Work out the finished part from the listing and answer in its coordinate system (mm). A direction names the side the tool comes from. Round coordinates to 2 decimals unless told otherwise and drop trailing zeros. Order: outer loops, then holes, each group sorted by start corner. A loop starts at its lowest first (then second) coordinate and runs counter-clockwise, first axis right, second up. Notation, with made-up numbers: (83.25, 31.5) - (107.25, 31.5) arc R5 ccw to (107.25, 39.5) - close; hole circle Ø9 at (87, -24.75). An arc over 180 degrees is marked (long way). Answer in a Markdown table with one row per item.
from build123d import *

# Parameters (mm, degrees)
SKETCH1_W               = 21
SKETCH1_H               = 4
SKETCH1_W_2             = 4
SKETCH1_R               = 1.5
BOSS_EXTRUDE1_DEPTH     = 2
SKETCH1_3_W             = 21
SKETCH1_3_H             = 4
BOSS_EXTRUDE2_DEPTH     = 40
CUT_EXTRUDE1_DEPTH      = 50.568134926
CUT_EXTRUDE1_DEPTH_BACK = 50.568134926


with BuildPart() as part:
    # Sketch1 → Boss-Extrude1 (new body)
    # profile 1 of 3: a face of its own
    with BuildSketch(Plane(origin=(0, 0, 0), x_dir=(1, 0, 0), z_dir=(0, 1, 0))):
        with Locations((14.5, 2)):
            Rectangle(SKETCH1_W, SKETCH1_H)
    # profile 2 of 3: a face of its own
    with BuildSketch(Plane(origin=(0, 0, 0), x_dir=(1, 0, 0), z_dir=(0, 1, 0))):
        with Locations((2, 2)):
            Rectangle(SKETCH1_W_2, SKETCH1_H)
        with Locations(Location((1.985523286, 2, 0), (0, 0, 270))):
            Circle(SKETCH1_R, mode=Mode.SUBTRACT)
    # profile 3 of 3: a face of its own
    with BuildSketch(Plane(origin=(0, 0, 0), x_dir=(1, 0, 0), z_dir=(0, 1, 0))):
        with Locations((27, 2)):
            Rectangle(SKETCH1_W_2, SKETCH1_H)
        with Locations(Location((26.985523286, 2, 0), (0, 0, 270))):
            Circle(SKETCH1_R, mode=Mode.SUBTRACT)
    extrude(amount=BOSS_EXTRUDE1_DEPTH)

    # Sketch1_3 → Boss-Extrude2 (add)
    with BuildSketch(Plane(origin=(0, 0, 0), x_dir=(1, 0, 0), z_dir=(0, 1, 0))):
        with Locations((14.5, 2)):
            Rectangle(SKETCH1_3_W, SKETCH1_3_H)
    extrude(amount=BOSS_EXTRUDE2_DEPTH)

    # Sketch4 → Cut-Extrude1 (cut, two sides: drawn at the far end of the back side and taken through both)
    with BuildSketch(Plane.XY.offset(-CUT_EXTRUDE1_DEPTH_BACK)):
        Polygon((14.829784235, 25.826592436), (15.580318165, 25.826592436), (15.580318165, 24.58059841), (17.192781023, 24.58059841), (19.245006478, 23.591132565), (19.245006478, 22.577235465), (17.982823566, 22.577235465), (17.650133225, 22.074575332), (18.051844448, 21.775593359), (18.251489115, 22.077235465), (19.444594864, 22.077235465), (21.728896307, 19.673543908), (21.340089812, 18.903582673), (21.919881884, 18.713869931), (22.47100439, 19.777672119), (19.745006478, 22.577235465), (19.745006478, 23.905142602), (17.307024063, 25.08059841), (16.080318165, 25.08059841), (16.080318165, 26.326592436), (14.829784235, 26.326592436), align=None)
        Polygon((13.027251973, 25.826592436), (13.917191226, 25.826592436), (13.917191226, 26.326592436), (12.527251973, 26.326592436), (12.527251973, 25.08059841), (11.339002885, 25.08059841), (8.862563659, 23.907548251), (8.862563659, 22.524621534), (6.115614244, 19.777672119), (6.67527171, 18.669699411), (7.27342553, 18.971837946), (6.874226368, 19.777672119), (9.208768581, 22.14696034), (10.304123515, 22.13906148), (10.411216966, 21.982171939), (10.824179507, 22.264061881), (10.56950065, 22.637160784), (9.362563659, 22.645864288), (9.362563659, 23.591132565), (11.451435998, 24.58059841), (13.027251973, 24.58059841), align=None)
        Polygon((17.834770022, 21.447616721), (17.428999134, 21.740464967), (16.875174702, 20.903694469), (15.097594277, 20.903694469), (15.097594277, 20.403694469), (16.97171728, 20.403694469), (18.980777312, 18.713869931), (17.724730843, 14.177305917), (19.569630531, 14.177305917), (21.712038769, 18.312681525), (21.136756911, 18.500918487), (19.245006478, 14.754647487), (18.482173443, 14.754647487), (19.745006478, 18.903582673), (17.415142863, 20.813604196), align=None)
        Polygon((11.752771943, 20.903694469), (11.07591062, 21.895281359), (10.662948079, 21.613391417), (11.249689352, 20.753828409), (8.862563659, 18.903582673), (10.041604324, 14.754647487), (9.362563659, 14.754647487), (7.428562862, 18.658673552), (6.830494871, 18.362398898), (8.952818152, 14.16076412), (10.833448813, 14.16076412), (9.629185319, 18.713869931), (11.691280342, 20.403694469), (13.634288417, 20.403694469), (13.634288417, 20.903694469), align=None)
    extrude(amount=CUT_EXTRUDE1_DEPTH + CUT_EXTRUDE1_DEPTH_BACK, mode=Mode.SUBTRACT)


solid = part.part
1) The mould has two halves that part along X. Classify faces 3 (the face through (29, 1, -2)), 4 (the face through (0, 1, -2)), 5 (the face through (19, 14.177, -2)): released by +X, released by -X, zero draft, split by the parting line, or undercut.
Filled in:
| item | result |
|---|---|
| face 3 | released by +X |
| face 4 | released by -X |
| face 5 | undercut |
2) Find the intervals of material crossed by probe 1 along Y at (x, z) = (12, -3.1); probe 2 along X at (y, z) = (0.8, -2); probe 3 along X at (y, z) = (23, -1.45) (3 decimals), in increasing order. Write a range as from..to.
Filled in:
| item | result |
|---|---|
| probe 1 | y = 0..20.4, 20.9..24.58, 25.08..40 |
| probe 2 | x = 0..0.49, 3.49..25.49, 28.49..29 |
| probe 3 | x = 4..8.863, 9.363..19.245, 19.745..25 |
3) Find section A-A, the plane z = -2. Give the number of separate pieces and of enclosed holes in the cut face, then the cut area to 3 significant figures.
Filled in:
| item | result |
|---|---|
| separate pieces | 3 |
| enclosed holes | 4 |
| area | 810 mm^2 |
4) Which of the six approach directions +Z, -Z, +X, -X, +Y, -Y give full straight-line access (tool end or side, diameter ignored) to faces 1 (the face through (13, 26.327, -2)), 2 (the face through (14, 0, -2))?
Filled in:
| item | result |
|---|---|
| face 1 | +Z, -Z |
| face 2 | +Z, -Z, +X, -X, -Y |
5) Find section B-B, the plane y = 35. Give the vertices of the cut face in (x, z).
Filled in:
| item | result |
|---|---|
| outline | (4, -4) - (25, -4) - (25, 0) - (4, 0) - close |
6) Each of these flat-tipped pins is pushed along its axis until it touches: pin 1 (1 mm diameter, centred on y = 25, z = -1.5, fed in from +X); pin 2 (1.2 mm diameter, centred on x = 2, z = -3, fed in from +Y). Where does it stop, or does it pass through?
Filled in:
| item | result |
|---|---|
| pin 1 | stops at x = 25 |
| pin 2 | stops at y = 2 |
